```python
from build123d import *

# Parameters (mm, degrees)
SKETCH1_R           = 12
SKETCH1_R_2         = 1.75
BOSS_EXTRUDE1_DEPTH = 9.5
SKETCH3_R           = 12
SKETCH3_R_2         = 9.5
BOSS_EXTRUDE2_DEPTH = 3
SKETCH4_R           = 1.3
CUT_EXTRUDE1_DEPTH  = 10.5
SKETCH5_W           = 10
SKETCH5_H           = 5
CUT_EXTRUDE2_DEPTH  = 3
FILLET1_R           = 0.5


with BuildPart() as part:
    # Sketch1 → Boss-Extrude1 (new body)
    with BuildSketch(Plane(origin=(0, 0, 0), x_dir=(1, 0, 0), z_dir=(0, 1, 0))):
        with BuildLine():
            Line((-17.857758621, 3.359755504), (-10.603448276, 10.609754222))
            ThreePointArc((-10.603448276, 10.609754222), (0, 15), (10.603448276, 10.609754222))
            Line((10.603448276, 10.609754222), (17.857758621, 3.359755504))
            ThreePointArc((17.857758621, 3.359755504), (19.25, 0), (17.857758621, -3.359755504))
            Line((17.857758621, -3.359755504), (10.603448276, -10.609754222))
            ThreePointArc((10.603448276, -10.609754222), (0, -15), (-10.603448276, -10.609754222))
            Line((-10.603448276, -10.609754222), (-17.857758621, -3.359755504))
            ThreePointArc((-17.857758621, -3.359755504), (-19.25, 0), (-17.857758621, 3.359755504))
        make_face()
        Circle(SKETCH1_R, mode=Mode.SUBTRACT)
        with Locations((-14.5, 0)):
            Circle(SKETCH1_R_2, mode=Mode.SUBTRACT)
        with Locations((14.5, 0)):
            Circle(SKETCH1_R_2, mode=Mode.SUBTRACT)
    extrude(amount=BOSS_EXTRUDE1_DEPTH)

    # Sketch3 → Boss-Extrude2 (add)
    with BuildSketch(Plane(origin=(0, 9.5, 0), x_dir=(1, 0, 0), z_dir=(0, 1, 0))):
        Circle(SKETCH3_R)
        Circle(SKETCH3_R_2, mode=Mode.SUBTRACT)
    extrude(amount=-BOSS_EXTRUDE2_DEPTH)

    # Sketch4 → Cut-Extrude1 (cut, through all)
    with BuildSketch(Plane(origin=(0, 9.5, 0), x_dir=(1, 0, 0), z_dir=(0, 1, 0))):
        with Locations((8.125, 8.125)):
            Circle(SKETCH4_R)
        with Locations((-8.125, 8.125)):
            Circle(SKETCH4_R)
        with Locations((-8.125, -8.125)):
            Circle(SKETCH4_R)
        with Locations((8.125, -8.125)):
            Circle(SKETCH4_R)
    extrude(amount=-CUT_EXTRUDE1_DEPTH, mode=Mode.SUBTRACT)

    # Sketch5 → Cut-Extrude2 (cut)
    with BuildSketch(Plane(origin=(0, 9.5, 0), x_dir=(1, 0, 0), z_dir=(0, 1, 0))):
        with Locations((0, -7.4)):
            Rectangle(SKETCH5_W, SKETCH5_H)
    extrude(amount=-CUT_EXTRUDE2_DEPTH, mode=Mode.SUBTRACT)

    # Fillet1
    fillet1_edges = [part.edges().sort_by_distance(p)[0] for p in [
        (-5, 8, 8.077747211),
        (5, 8, 8.077747211),
        (-5, 8, 9.9),
        (5, 8, 9.9),
    ]]
    fillet(fillet1_edges, radius=FILLET1_R)


solid = part.part
```
Geometry: final body of the model. Coordinates: model frame, mm. A direction names the side the tool comes from. Coordinates: 2 decimals unless noted, no trailing zeros. Order: outer loops, then holes, each group sorted by start corner. A loop starts at its lowest first (then second) coordinate and runs counter-clockwise, first axis right, second up. Notation, with made-up numbers: (20.25, 38.5) - (55.25, 38.5) arc R23 cw to (55.25, 63.5) - close; hole circle Ø5 at (57.25, 67.25). An arc over 180 degrees is marked (long way). Return JSON: item names as keys, results as strings. Group by question number.
1. Cut plane B-B (z = -4). Output: boundary loops of the cut face in (x, y), plus the area to 3 significant figures.
2. Set-up query: faces 4 (the face through (0, 3, 12)), 5 (the face through (-14.18, 4.684, 7.036)). Return all of +Z, -Z, +X, -X, +Y, -Y with unobstructed straight access to the full face (end or side cutting, diameter ignored); none if empty.
3. Pull-direction query (Z, two-part tool) for faces 1 (the face through (0, 5, -15)), 2 (the face through (-19.25, 4.68, 0.05)), 3 (the face through (16.169, 4.684, -0.526)); classes: pulls with the +Z half, pulls with the -Z half, needs draft (parallel to the pull), parting line crosses it, or undercut.
4. Cut plane A-A (x = 0). Output: boundary loops of the cut face in (y, z).
5. Cut plane D-D (y = 7.25). Output: boundary loops of the cut face in (x, z) (3 decimals), plus the area to 3 significant figures.
6. Material intervals for line 1 along Z through (x, y) = (0, 7.9); line 2 along Z through (x, y) = (1, 9); line 3 along Y through (x, z) = (-0.5, -10.5), sorted ascending. Write a range as [from, to].
7. Cut plane C-C (y = 5.25). Output: boundary loops of the cut face in (x, z) (3 decimals).
8. Pin query (flat end, axial travel): pin 1 (2 mm diameter, centred on x = -6, y = 8.5, fed in from -Z); pin 2 (2.5 mm diameter, centred on x = 0.5, y = 8.5, fed in from -Z); pin 3 (2 mm diameter, centred on x = -3, y = 2.5, fed in from +Z); pin 4 (4 mm diameter, centred on x = -10, y = 1, fed in from +Z). Return the tip coordinate at first contact, or that it passes through.
Resolved:
{
 "1": {"outline": "(-17.22, 0) - (-11.31, 0) - (-11.31, 6.5) - (-8.62, 6.5) - (-8.62, 9.5) - (-17.22, 9.5) - close; (8.62, 6.5) - (11.31, 6.5) - (11.31, 0) - (17.22, 0) - (17.22, 9.5) - (8.62, 9.5) - close", "area": "128 mm²"},
 "2": {"face 4": "-Y", "face 5": "+Z, -X, +Y, -Y"},
 "3": {"face 1": "pulls with the -Z half", "face 2": "parting line crosses it", "face 3": "undercut"},
 "4": {"outline": "(0, -15) - (9.5, -15) - (9.5, -9.5) - (6.5, -9.5) - (6.5, -12) - (0, -12) - close; (0, 12) - (6.5, 12) - (6.5, 9.9) - (9.5, 9.9) - (9.5, 15) - (0, 15) - close"},
 "5": {"outline": "(-17.858, -3.36) - (-10.603, -10.61) arc R15 ccw to (10.603, -10.61) - (17.858, -3.36) arc R4.75 ccw to (17.858, 3.36) - (10.603, 10.61) arc R15 ccw to (-10.603, 10.61) - (-17.858, 3.36) arc R4.75 ccw to start; hole circle Ø3.5 at (-14.5, 0); hole circle Ø2.6 at (-8.125, -8.125); hole circle Ø2.6 at (-8.125, 8.125); hole (-5.225, 7.934) arc R9.5 ccw (long way) to (5.225, 7.934) arc R0.5 cw to (5, 8.352) - (5, 9.4) arc R0.5 ccw to (4.5, 9.9) - (-4.5, 9.9) arc R0.5 ccw to (-5, 9.4) - (-5, 8.352) arc R0.5 cw to start; hole circle Ø2.6 at (8.125, -8.125); hole circle Ø2.6 at (8.125, 8.125); hole circle Ø3.5 at (14.5, 0)", "area": "461 mm²"},
 "6": {"line 1": "z = [-15, -9.5], [9.9, 15]", "line 2": "z = [-14.97, -9.45], [9.9, 14.97]", "line 3": "y = [6.5, 9.5]"},
 "7": {"outline": "(-17.858, -3.36) - (-10.603, -10.61) arc R15 ccw to (10.603, -10.61) - (17.858, -3.36) arc R4.75 ccw to (17.858, 3.36) - (10.603, 10.61) arc R15 ccw to (-10.603, 10.61) - (-17.858, 3.36) arc R4.75 ccw to start; hole circle Ø3.5 at (-14.5, 0); hole (-9.304, -7.578) arc R1.3 ccw to (-7.578, -9.304) arc R12 ccw to (7.578, -9.304) arc R1.3 ccw to (9.304, -7.578) arc R12 ccw to (9.304, 7.578) arc R1.3 ccw to (7.578, 9.304) arc R12 ccw to (-7.578, 9.304) arc R1.3 ccw to (-9.304, 7.578) arc R12 ccw to start; hole circle Ø3.5 at (14.5, 0)"},
 "8": {"pin 1": "stops at z = -14.14", "pin 2": "stops at z = -15", "pin 3": "stops at z = 14.87", "pin 4": "stops at z = 12.69"}
}
